Source: CAD feature listing. Evaluate the final solid. Frame: model axes, mm. A direction names the side the tool comes from. Give positions to 0.01 mm unless a question says otherwise; leave off trailing zeros. Order: outer loops, then holes, each group sorted by start corner. A loop starts at its lowest first (then second) coordinate and runs counter-clockwise, first axis right, second up.
from build123d import *

# Parameters (mm, degrees)
SKETCH1_W           = 40
SKETCH1_H           = 30
BOSS_EXTRUDE1_DEPTH = 20
BOSS_EXTRUDE2_DEPTH = 4
SKETCH4_R           = 2.5
CUT_EXTRUDE1_DEPTH  = 5


with BuildPart() as part:
    # Sketch1 → Boss-Extrude1 (new body)
    with BuildSketch(Plane.XY):
        Rectangle(SKETCH1_W, SKETCH1_H)
    extrude(amount=-BOSS_EXTRUDE1_DEPTH)

    # Sketch3 → Boss-Extrude2 (add)
    with BuildSketch(Plane(origin=(0, 15, 0), x_dir=(1, 0, 0), z_dir=(0, 1, 0))):
        with BuildLine():
            Line((-12.97722879, 13.914589169), (-3.400294542, 11.921916457))
            ThreePointArc((-3.400294542, 11.921916457), (-1.837109147, 10), (-3.400294542, 8.078083543))
            Line((-3.400294542, 8.078083543), (-12.97722879, 6.085410831))
            ThreePointArc((-12.97722879, 6.085410831), (-17.790166122, 10), (-12.97722879, 13.914589169))
        make_face()
        with BuildLine():
            Line((-13.18093595, 12.935557304), (-3.604001703, 10.942884592))
            ThreePointArc((-3.604001703, 10.942884592), (-2.837109147, 10), (-3.604001703, 9.057115408))
            Line((-3.604001703, 9.057115408), (-13.18093595, 7.064442696))
            ThreePointArc((-13.18093595, 7.064442696), (-16.790166122, 10), (-13.18093595, 12.935557304))
        make_face(mode=Mode.SUBTRACT)
    extrude(amount=BOSS_EXTRUDE2_DEPTH)

    # Sketch4 → Cut-Extrude1 (cut)
    with BuildSketch(Plane(origin=(0, 15, 0), x_dir=(1, 0, 0), z_dir=(0, 1, 0))):
        with Locations(Location((-13.791737359, 10, 0), (0, 0, 270))):
            Circle(SKETCH4_R)
    extrude(amount=-CUT_EXTRUDE1_DEPTH, mode=Mode.SUBTRACT)


solid = part.part
1) Section query A-A on z = -10. Output: boundary loops of the cut face in (x, y), and give its area (3 significant figures).
Checks:
outline: (-20, -15) - (20, -15) - (20, 15) - (-1.84, 15) - (-1.84, 19) - (-2.84, 19) - (-2.84, 15) - (-11.29, 15) - (-11.29, 10) - (-16.29, 10) - (-16.29, 15) - (-16.79, 15) - (-16.79, 19) - (-17.79, 19) - (-17.79, 15) - (-20, 15) - close
area: 1,180 mm2
2) Section query D-D on z = -3.5. Output: boundary loops of the cut face in (x, y), and give its area (3 significant figures).
Checks:
outline: (-20, -15) - (20, -15) - (20, 15) - (-20, 15) - close
area: 1,200 mm2
3) Pull-direction query (Z, two-part tool) for faces 1 (the face through (-2.837, 16.972, -10.018)), 2 (the face through (0, -15, -10)), 3 (the face through (-17.79, 16.97, -9.9)); classes: +Z half, -Z half, draft (parallel to the pull), parting line (faces both ways), or undercut.
Checks:
face 1: undercut
face 2: draft
face 3: parting line
4) Section query C-C on x = -12. Output: boundary loops of the cut face in (y, z), and give its area (3 significant figures).
Checks:
outline: (-15, -20) - (15, -20) - (15, -13.71) - (19, -13.71) - (19, -12.69) - (15, -12.69) - (15, -11.74) - (10, -11.74) - (10, -8.26) - (15, -8.26) - (15, -7.31) - (19, -7.31) - (19, -6.29) - (15, -6.29) - (15, 0) - (-15, 0) - close
area: 591 mm2
5) Ray query, L1, parallel to X at y = 17.55, z = -10; L2, parallel to X at y = 13, z = -10; L3, parallel to Y at x = -17, z = -3.5. Return the intervals inside material, ascending.
Checks:
L1: x = -17.79 to -16.79, -2.84 to -1.84
L2: x = -20 to -16.29, -11.29 to 20
L3: y = -15 to 15
6) Reachability of faces 4 (the face through (-8.1, 17, -7.1)), 5 (the face through (-8.256, 16.972, -12.932)), 6 (the face through (-1.837, 16.972, -10.038)), 7 (the face through (-12.1, 12.54, -11.84)) from +Z, -Z, +X, -X, +Y, -Y: full face, straight path, thin tool, end or side. Return the list, or none.
Checks:
face 4: +Z, +X, +Y
face 5: -Z, +X, +Y
face 6: +X, +Y
face 7: +Y
7) First-contact query: pin 1 Ø5 at (x, z) = (1, -14.5) entering from +Y; pin 2 Ø2.5 at (x, z) = (-14.5, -10.5) entering from +Y. Flat tips, straight axial feed; report the tip coordinate or a pass-through.
Checks:
pin 1: stops at y = 15
pin 2: stops at y = 10
8) Section query B-B on x = -6.5. Output: boundary loops of the cut face in (y, z), and give its area (3 significant figures).
Checks:
outline: (-15, -20) - (15, -20) - (15, -12.57) - (19, -12.57) - (19, -11.55) - (15, -11.55) - (15, -8.45) - (19, -8.45) - (19, -7.43) - (15, -7.43) - (15, 0) - (-15, 0) - close
area: 608 mm2
